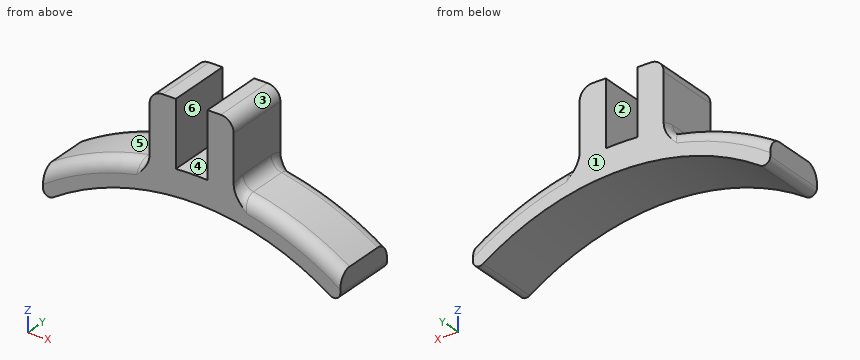
Autodesk Inventor part; units mm, degrees
ref_plane "YZ Plane" through (0, 0, 0) normal (1, 0, 0) x (0, 1, 0)
ref_plane "XZ Plane" through (0, 0, 0) normal (0, 1, 0) x (-1, 0, 0)
sketch "스케치1" plane through (0, 0, 0) normal (0, 1, 0) x (-1, 0, 0)
  line L0 (-6.5, -10) -> (-6.5, 10)
  line L1 (6.5, 10) -> (6.5, -10)
  line L2 (6.5, -10) -> (-6.5, 10) construction
  line L3 (-6.5, -10) -> (6.5, 10) construction
  line L4 (2.45, -10) -> (-2.45, -10)
  line L5 (-2.45, -10) -> (-2.45, 10)
  line L6 (-2.45, 10) -> (2.45, 10)
  line L7 (2.45, 10) -> (2.45, -10)
  line L8 (2.45, -10) -> (-2.45, 10) construction
  line L9 (-2.45, -10) -> (2.45, 10) construction
  arc A0 (22.9827, -6.6573) -> (-22.9827, -6.6573) centre (0, -43) ccw
  arc A1 (22.9827, -11.4914) -> (-22.9827, -11.4914) centre (0, -43) ccw
  line L10 (22.9827, -11.4914) -> (22.9827, -6.6573)
  line L11 (-22.9827, -11.4914) -> (-22.9827, -6.6573)
  line L12 (-6.5, 10) -> (-2.45, 10)
  line L13 (2.45, 10) -> (6.5, 10)
  line L14 (6.5, -10) -> (2.45, -10)
  line L15 (-2.45, -10) -> (-6.5, -10)
  point P0 (0, 0)
  point P1 (6.5, -0.4941)
  point P2 (2.45, -0.0699)
  point P3 (-2.45, -0.0699)
  point P4 (-6.5, -0.4941)
  dimension "d0" = 13
  dimension "d1" = 20
  dimension "d2" = 4.9
  dimension "d3" = 86
  dimension "d4" = 4
sketch "스케치2" plane through (0, 0, 0) normal (0, 0, 1) x (1, 0, 0)
  point P0 (0, 0)
ref_plane "작업 평면1" through (0, 0, -43) normal (0, 0, 1) x (1, 0, 0)
sketch "스케치3" plane through (0, 0, -43) normal (0, 0, 1) x (1, 0, 0)
  line L0 (0, 0) -> (-26.5437, 0)
  line L1 (-26.5437, 0) -> (31.7273, 0)
extrude "돌출1" add sketch "스케치1" along normal blind 10 contours A1 L11 A0 L0 | L0 A0 L5 A1 | L0 L12 L5 A0 | L5 A0 L7 A1 | L7 A0 L1 A1 | L7 L13 L1 A0 | L1 A0 L10 A1
fillet "모깎기2" radius 1 2 edges at (22.9827, 5, -11.4914) (-22.9827, 5, -11.4914)
fillet "모깎기3" radius 2 6 edges at (-15.06, 0, -2.7235) (15.06, 0, -2.7235) (15.06, 10, -2.7235) (-15.06, 10, -2.7235) (6.5, 5, 10) (-6.5, 5, 10)
fillet "모깎기4" radius 2 2 edges at (-6.5, 5, -0.4941) (6.5, 5, -0.4941)
properties part number "날개꼽는파트"
Work out the finished part from the listing and answer in its coordinate system (mm). Face numbers are marked on the shaded views. A direction names the side the tool comes from. Give positions to 0.01 mm unless a question says otherwise; leave off trailing zeros. Write each loop counter-clockwise with the first axis right and the second up, starting at its lowest first coordinate (ties: lowest second). Pieces come first, ordered by that corner, then holes.
Q1. A tool of negligible diameter and unlimited length cuts with its end or side. For the marked faces 1 and 2, from which of +Z, -Z, +X, -X, +Y, -Y can it reach the whole face along a straight path? Write none if from no direction.
Answer:
face 1: +Z, -Z, +X, -X, +Y
face 2: +Z, +Y, -Y
Q2. Straight lines are drawn through the part: L1, parallel to X at y = 3.5, z = 4.75; L2, parallel to X at y = 1.25, z = -7; L3, parallel to Z at x = 0.5, y = 8.75. For each, find the intervals that lie inside material, in ascending order.
Answer:
L1: x = -6.5 to -2.45, 2.45 to 6.5
L2: x = -22.98 to -15, 15 to 22.98
L3: z = -4 to 0
Q3. The part is cut by section A-A on y = 4. Give the vertices of the cut face in (x, z).
Answer:
outline: (-22.98, -9.58) arc R1 ccw to (-21.43, -10.42) arc R39 cw to (21.43, -10.42) arc R1 ccw to (22.98, -9.58) - (22.98, -6.66) arc R43 ccw to (8.12, -0.77) arc R2 cw to (6.5, 1.19) - (6.5, 8) arc R2 ccw to (4.5, 10) - (2.45, 10) - (2.45, -0.07) arc R43 ccw to (-2.45, -0.07) - (-2.45, 10) - (-4.5, 10) arc R2 ccw to (-6.5, 8) - (-6.5, 1.19) arc R2 cw to (-8.12, -0.77) arc R43 ccw to (-22.98, -6.66) - close
Q4. Given pin 1 (3.5 mm diameter, centred on y = 4, z = 2.5, fed in from -X); pin 2 (10 mm diameter, centred on x = 5.5, z = 6, fed in from -Y); pin 3 (1.5 mm diameter, centred on x = -13.5, y = 4, fed in from +Z); pin 4 (2 mm diameter, centred on y = 1, z = 1, fed in from -X), each flat-ended and moving along its own axis, determine where each tip first touches the part or whether it passes through.
Answer:
pin 1: stops at x = -6.55
pin 2: stops at y = 0
pin 3: stops at z = -1.93
pin 4: stops at x = -6.81
Q5. The part is cut by section C-C on x = 3.5. Give the vertices of the cut face in (y, z), and give its area (3 significant figures).
Answer:
outline: (0, -4.16) - (10, -4.16) - (10, 10) - (0, 10) - close
area: 142 mm2
Q6. The part is cut by section B-B on x = -5.5. Give the vertices of the cut face in (y, z).
Answer:
outline: (0, -4.39) - (10, -4.39) - (10, 9.73) - (0, 9.73) - close
Q7. For a pull along X with two mould halves and no side action, classify the marked faces 3, 4, 5 and 6 as released by +X, released by -X, zero draft, split by the parting line, or undercut.
Answer:
face 3: released by +X
face 4: undercut
face 5: released by -X
face 6: undercut
